from build123d import *

# Parameters (mm, degrees)
PAD004_DEPTH            = 102
SKETCH006_R             = 2.75
POCKET001_DEPTH         = 19.3215080757
SKETCH007_R             = 5
POCKET002_DEPTH         = 14.3215080757
BODY002_PLACEMENT_ANGLE = 180


with BuildPart() as part:
    # Sketch004 → Pad004 (new body)
    with BuildSketch(Plane.YZ):
        Polygon((-5.5, 4), (-5.5, 20.4544826719), (-10.5, 20.4544826719), (-20, 4), (-20, 0), (0, 0), (0, 4), align=None)
    extrude(amount=-PAD004_DEPTH)

    # Sketch006 (on Face3 of Pad004) → Pocket001 (cut, through all)
    with BuildSketch(Plane(origin=(0, -16.7320508076, 9.6602540378), x_dir=(0, -0.5, -0.8660254038), z_dir=(0, -0.8660254038, 0.5))):
        with Locations((-3.4641016151, -31.95)):
            Circle(SKETCH006_R)
        with Locations((-3.4641016151, -70.05)):
            Circle(SKETCH006_R)
    extrude(amount=-POCKET001_DEPTH, mode=Mode.SUBTRACT)

    # Sketch007 (on Face10 of Pocket001) → Pocket002 (cut, through all)
    with BuildSketch(Plane(origin=(0, -12.4019237886, 7.1602540378), x_dir=(0, -0.5, -0.8660254038), z_dir=(0, -0.8660254038, 0.5))):
        with Locations((-3.4641016151, -31.95)):
            Circle(SKETCH007_R)
        with Locations((-3.4641016151, -70.05)):
            Circle(SKETCH007_R)
    extrude(amount=-POCKET002_DEPTH, mode=Mode.SUBTRACT)


with BuildPart() as part_1:
    # Body002 placement: moved
    add(part.part.moved(Location((2, 35, 36))).rotate(Axis((2, 35, 36), (0, 0, 1)), BODY002_PLACEMENT_ANGLE))


solid = part_1.part
For this review, take the finished solid that the model builds, in its own axes (mm). A direction names the side the tool comes from. Give positions to 0.01 mm unless a question says otherwise; leave off trailing zeros. Order: outer loops, then holes, each group sorted by start corner. A loop starts at its lowest first (then second) coordinate and runs counter-clockwise, first axis right, second up. Notation, with made-up numbers: (-35, -11.5) - (-11, -11.5) arc R19 ccw to (-11, 16.5) - close; hole circle Ø2 at (26.25, 81). An arc over 180 degrees is marked (long way). Answer as a JSON object with one key per item and string values. Group by question number.
Item 1: Machinability: for faces 1 (the flat face through (90, 38, 40)), 2 (the flat face through (104, 45, 44)), 3 (the flat face through (74.202, 46.746, 44.296)), which of the approach directions +Z, -Z, +X, -X, +Y, -Y give a long, thin tool a straight path to every point of the face, cutting with its end or side? Answer none if there is none.
Item 2: Clearance check with flat-ended pins moving along their axes: pin 1 Ø1 at (x, z) = (82.5, 52) entering from -Y; pin 2 Ø3 at (x, y) = (16, 38.5) entering from +Z; pin 3 Ø1.5 at (x, z) = (42, 41) entering from +Y. State where each tip first meets the part, or that it passes through.
Item 3: Wall thickness on line 1 along X through (y, z) = (37.5, 37); line 2 along X through (y, z) = (48.5, 49.5); line 3 along Z through (x, y) = (30, 42.5): over which ranges is each line inside the solid? List them lowest first.
Item 4: Take a section at D-D on y = 52.5. Give the boundary of the cut face in (x, z).
Item 5: Take a section at A-A on x = 27.5. Give the boundary of the cut face in (y, z), and give its area (3 significant figures).
Item 6: Take a section at B-B on y = 36.5. Give the number of separate pieces and of enclosed holes in the cut face, and give its area (3 significant figures).
Item 7: Draft analysis for pull direction Y (two halves, no side actions). For faces 4 (the flat face through (16, 38, 40)), 5 (the flat face through (36.102, 46.746, 44.296)), 6 (the flat face through (16, 35, 38)), state which applies: pulls with the +Y half, pulls with the -Y half, needs draft (parallel to the pull), parting line crosses it, or undercut.
Reported:
{
 "1": {"face 1": "+Z, +X, -X, -Y", "face 2": "+Z, -Z, +X, +Y, -Y", "face 3": "none"},
 "2": {"pin 1": "y = 40.5", "pin 2": "z = 40", "pin 3": "y = 54.86"},
 "3": {"line 1": "2 to 30.76, 37.14 to 68.86, 75.24 to 104", "line 2": "2 to 31.63, 36.27 to 69.73, 74.37 to 104", "line 3": "36 to 40.79, 47.87 to 56.45"},
 "4": {"outline": "(2, 36) - (104, 36) - (104, 44.33) - (2, 44.33) - close"},
 "5": {"outline": "(35, 36) - (55, 36) - (55, 40) - (45.5, 56.45) - (40.5, 56.45) - (40.5, 40) - (35, 40) - close", "area": "240 mm^2"},
 "6": {"separate pieces": "3", "enclosed holes": "0", "area": "341 mm^2"},
 "7": {"face 4": "needs draft", "face 5": "undercut", "face 6": "pulls with the -Y half"}
}
